For this review, take the finished solid that the model builds, in its own axes (mm). A direction names the side the tool comes from. Give positions to 0.01 mm unless a question says otherwise; leave off trailing zeros. Write each loop counter-clockwise with the first axis right and the second up, starting at its lowest first coordinate (ties: lowest second). Pieces come first, ordered by that corner, then holes.
1) For P1, Ø10, axis at y = 97, z = 26, coming from the +X side; P2, Ø3, axis at x = -8, y = 40, coming from the -Z side; P3, Ø9, axis at x = -3, y = 66, coming from the +Z side, all flat-tipped, find the tip position at first contact; note any pin that passes through.
2) We need section A-A on z = 0. Give the boundary of the cut face in (x, y).
3) Machinability: for faces 1 (the face through (-15, 73, 0)), 2 (the face through (39.65, 86.654, 3.461)), 3 (the face through (0, 55, -34.871)), which of the approach directions +Z, -Z, +X, -X, +Y, -Y give a long, thin tool a straight path to every point of the face, cutting with its end or side? Answer none if there is none.
4) We need section C-C on y = 16.5. Give the boundary of the cut face in (x, z).
5) We need section D-D on z = 16. Give the boundary of the cut face in (x, y).
6) We need section B-B on x = 7.5. Give the boundary of the cut face in (y, z).
7) Wall thickness on line 1 along X through (y, z) = (31.5, 32.5); line 2 along X through (y, z) = (12.5, 34); line 3 along Z through (x, y) = (5, 56): over which ranges is each line inside the solid? List them lowest first.
from build123d import *

# Parameters (mm, degrees)
SKETCH1_W           = 50
SKETCH1_H           = 100
BOSS_EXTRUDE1_DEPTH = 30
SKETCH3_W           = 30
SKETCH3_H           = 69.741989622
BOSS_EXTRUDE2_DEPTH = 50
SKETCH4_R           = 34.693390841
BOSS_EXTRUDE3_DEPTH = 30
SKETCH6_R           = 7.5
BOSS_EXTRUDE4_DEPTH = 50


with BuildPart() as part:
    # Sketch1 → Boss-Extrude1 (new body)
    with BuildSketch(Plane(origin=(0, 0, 0), x_dir=(1, 0, 0), z_dir=(0, 1, 0))):
        Rectangle(SKETCH1_W, SKETCH1_H)
    extrude(amount=BOSS_EXTRUDE1_DEPTH)

    # Sketch3 → Boss-Extrude2 (add)
    with BuildSketch(Plane(origin=(0, 30, 0), x_dir=(1, 0, 0), z_dir=(0, 1, 0))):
        Rectangle(SKETCH3_W, SKETCH3_H)
    extrude(amount=BOSS_EXTRUDE2_DEPTH)

    # Sketch4 → Boss-Extrude3 (add)
    with BuildSketch(Plane(origin=(15, 0, 0), x_dir=(0, 0, -1), z_dir=(1, 0, 0))):
        with Locations((0, 80)):
            Circle(SKETCH4_R)
    extrude(amount=-BOSS_EXTRUDE3_DEPTH)

    # Sketch6 → Boss-Extrude4 (add)
    with BuildSketch(Plane(origin=(15, 0, 0), x_dir=(0, 0, -1), z_dir=(1, 0, 0))):
        with Locations(Location((0, 80, 0), (0, 0, 180))):
            Circle(SKETCH6_R)
    extrude(amount=BOSS_EXTRUDE4_DEPTH)


solid = part.part
Results list:
1. P1: stops at x = 15
1. P2: stops at z = -34.87
1. P3: stops at z = 34.87
2. outline: (-25, 0) - (25, 0) - (25, 30) - (15, 30) - (15, 72.5) - (65, 72.5) - (65, 87.5) - (15, 87.5) - (15, 114.69) - (-15, 114.69) - (-15, 30) - (-25, 30) - close
3. face 1: +Z, -Z, -X, +Y
3. face 2: +X
3. face 3: -Z, +X, -X, +Y
4. outline: (-25, -50) - (25, -50) - (25, 50) - (-25, 50) - close
5. outline: (-25, 0) - (25, 0) - (25, 30) - (15, 30) - (15, 110.78) - (-15, 110.78) - (-15, 30) - (-25, 30) - close
6. outline: (0, -50) - (30, -50) - (30, -34.87) - (80, -34.87) - (80, -34.69) arc R34.69 ccw to (80, 34.69) - (80, 34.87) - (30, 34.87) - (30, 50) - (0, 50) - close
7. line 1: x = -15 to 15
7. line 2: x = -25 to 25
7. line 3: z = -34.87 to 34.87
